from build123d import *

# Parameters (mm, degrees)
ESQUISSE1_W        = 400
ESQUISSE1_H        = 400
ESQUISSE1_R        = 150
BOSS_EXTRU_1_DEPTH = 5
BOSS_EXTRU_2_START = -5
BOSS_EXTRU_2_DEPTH = 5
BOSS_EXTRU_4_START = -5
BOSS_EXTRU_4_DEPTH = 5


with BuildPart() as part:
    # Esquisse1 → Boss.-Extru.1 (new body)
    with BuildSketch(Plane.XY):
        Rectangle(ESQUISSE1_W, ESQUISSE1_H)
        Circle(ESQUISSE1_R, mode=Mode.SUBTRACT)
    extrude(amount=BOSS_EXTRU_1_DEPTH)

    # Esquisse2 → Boss.-Extru.2 (add)
    with BuildSketch(Plane.XY.offset(5).offset(BOSS_EXTRU_2_START)):
        with BuildLine():
            ThreePointArc((-66.275928016, -134.564116188), (17.903034415, -98.409800426), (109.421717045, -102.600622995))
            ThreePointArc((109.421717045, -102.600622995), (26.84783049, -147.57775577), (-66.275928016, -134.564116188))
        make_face()
    extrude(amount=BOSS_EXTRU_2_DEPTH)

    # Esquisse5 → Boss.-Extru.4 (add)
    with BuildSketch(Plane.XY.offset(5).offset(BOSS_EXTRU_4_START)):
        with BuildLine():
            Line((-18.866345265, -83.351919662), (-20.37407273, -83.74523987))
            add(Edge.make_bspline(
                [(-20.37407273, -83.74523987), (-18.831576298, -81.763764071), (-16.735860805, -80.369241418)],
                knots=[0, 0, 0, 1, 1, 1], degree=2))
            add(Edge.make_bspline(
                [(-16.735860805, -80.369241418), (-19.802386047, -79.615782741), (-22.460949022, -81.422874022)],
                knots=[0, 0, 0, 1, 1, 1], degree=2))
            Line((-22.460949022, -81.422874022), (-21.677782316, -79.558228062))
            add(Edge.make_bspline(
                [(-21.677782316, -79.558228062), (-24.26181325, -80.142481289), (-25.822525036, -82.262094558)],
                knots=[0, 0, 0, 1, 1, 1], degree=2))
            Line((-25.822525036, -82.262094558), (-25.822525036, -81.483648674))
            add(Edge.make_bspline(
                [(-25.822525036, -81.483648674), (-28.351333433, -83.259460466), (-29.053841556, -86.259564776)],
                knots=[0, 0, 0, 1, 1, 1], degree=2))
            Line((-29.053841556, -86.259564776), (-29.496527169, -84.468232294))
            add(Edge.make_bspline(
                [(-29.496527169, -84.468232294), (-30.385431001, -86.732906367), (-30.059960229, -91.485672478), (-26.658406188, -96.353832625), (-25.176717422, -99.770059496), (-25.385021469, -101.387375039)],
                knots=[0, 0, 0, 0, 0.406589929, 0.730891559, 1, 1, 1, 1], degree=3))
            add(Edge.make_bspline(
                [(-25.385021469, -101.387375039), (-26.802377477, -98.375380833), (-29.974054698, -97.359243335)],
                knots=[0, 0, 0, 1, 1, 1], degree=2))
            Line((-29.974054698, -97.359243335), (-32.122945451, -94.451438986))
            Line((-32.122945451, -94.451438986), (-30.527430237, -94.731681614))
            Line((-30.527430237, -94.731681614), (-31.880933057, -92.683136884))
            Line((-31.880933057, -92.683136884), (-33.497007064, -90.538320458))
            Line((-33.497007064, -90.538320458), (-32.581262202, -90.538320458))
            Line((-32.581262202, -90.538320458), (-33.613359396, -89.007007118))
            Line((-33.613359396, -89.007007118), (-36.217522242, -87.522991031))
            Line((-36.217522242, -87.522991031), (-34.976085707, -87.301815556))
            Line((-34.976085707, -87.301815556), (-36.099822643, -86.512016486))
            add(Edge.make_bspline(
                [(-36.099822643, -86.512016486), (-39.217212358, -85.557948169), (-40.645373336, -82.598959987)],
                knots=[0, 0, 0, 1, 1, 1], degree=2))
            add(Edge.make_bspline(
                [(-40.645373336, -82.598959987), (-39.03359815, -80.653112191), (-34.181178142, -77.850858673), (-32.852259513, -72.300227157), (-30.904376568, -70.414710171)],
                knots=[0, 0, 0, 0, 0.487449068, 1, 1, 1, 1], degree=3))
            Line((-30.904376568, -70.414710171), (-31.646902368, -69.877944585))
            Line((-31.646902368, -69.877944585), (-29.609451058, -70.166012753))
            Line((-29.609451058, -70.166012753), (-30.237434638, -69.028235393))
            Line((-30.237434638, -69.028235393), (-32.249484484, -67.755751936))
            Line((-32.249484484, -67.755751936), (-30.841080327, -67.755751936))
            Line((-30.841080327, -67.755751936), (-32.866048633, -66.115953665))
            Line((-32.866048633, -66.115953665), (-32.122945451, -65.705806115))
            Line((-32.122945451, -65.705806115), (-34.976085707, -62.978029277))
            add(Edge.make_bspline(
                [(-34.976085707, -62.978029277), (-34.102733297, -60.394072595), (-33.737935509, -52.117151528), (-39.05614256, -45.345642181), (-42.031693147, -41.294166441)],
                knots=[0, 0, 0, 0, 0.344230119, 1, 1, 1, 1], degree=3))
            Line((-42.031693147, -41.294166441), (-43.185854427, -41.294166441))
            Line((-43.185854427, -41.294166441), (-44.096631121, -43.298315386))
            add(Edge.make_bspline(
                [(-44.096631121, -43.298315386), (-45.231201574, -46.338252094), (-48.330686607, -50.268996334), (-48.834287807, -55.064729459), (-49.3765867, -56.376310655)],
                knots=[0, 0, 0, 0, 0.699335622, 1, 1, 1, 1], degree=3))
            add(Edge.make_bspline(
                [(-49.3765867, -56.376310655), (-53.035018211, -56.310042975), (-56.717874117, -57.429335725), (-59.748293818, -59.471450261)],
                knots=[0, 0, 0, 0, 1, 1, 1, 1], degree=3))
            add(Edge.make_bspline(
                [(-59.748293818, -59.471450261), (-61.730136737, -57.382399641), (-67.02409653, -54.780846239), (-72.769327351, -53.559543058), (-75.231721344, -51.783479704)],
                knots=[0, 0, 0, 0, 0.486790351, 1, 1, 1, 1], degree=3))
            Line((-75.231721344, -51.783479704), (-76.616603351, -52.328679392))
            Line((-76.616603351, -52.328679392), (-76.910233832, -52.974808375))
            add(Edge.make_bspline(
                [(-76.910233832, -52.974808375), (-76.187929468, -60.035339336), (-73.946183278, -67.404517716), (-68.30337696, -72.2011591)],
                knots=[0, 0, 0, 0, 1, 1, 1, 1], degree=3))
            Line((-68.30337696, -72.2011591), (-70.400668481, -77.268167724))
            Line((-70.400668481, -77.268167724), (-70.400668481, -78.023881232))
            Line((-70.400668481, -78.023881232), (-69.598297697, -77.87343671))
            Line((-69.598297697, -77.87343671), (-70.283656075, -80.205357998))
            Line((-70.283656075, -80.205357998), (-70.283656075, -80.865611092))
            Line((-70.283656075, -80.865611092), (-69.087412979, -80.205357998))
            Line((-69.087412979, -80.205357998), (-69.721157599, -81.884742883))
            Line((-69.721157599, -81.884742883), (-69.721157599, -83.255626103))
            Line((-69.721157599, -83.255626103), (-68.175660205, -82.19091787))
            Line((-68.175660205, -82.19091787), (-68.497334605, -83.74523987))
            Line((-68.497334605, -83.74523987), (-67.932636696, -83.958338287))
            add(Edge.make_bspline(
                [(-67.932636696, -83.958338287), (-65.874908009, -84.443832393), (-61.558935468, -86.72875783), (-56.654005751, -85.685370072), (-54.241439725, -85.638363098)],
                knots=[0, 0, 0, 0, 0.460172434, 1, 1, 1, 1], degree=3))
            add(Edge.make_bspline(
                [(-54.241439725, -85.638363098), (-53.550315945, -86.398092796), (-52.60563993, -89.456662165), (-54.737135432, -92.036882428), (-55.189595432, -93.773610113)],
                knots=[0, 0, 0, 0, 0.354288348, 1, 1, 1, 1], degree=3))
            Line((-55.189595432, -93.773610113), (-54.110273533, -93.367103715))
            Line((-54.110273533, -93.367103715), (-55.189595432, -95.920472028))
            Line((-55.189595432, -95.920472028), (-55.189595432, -98.016520642))
            Line((-55.189595432, -98.016520642), (-54.649934483, -97.457574345))
            Line((-54.649934483, -97.457574345), (-54.919764957, -99.950163153))
            Line((-54.919764957, -99.950163153), (-54.649934483, -102.693612698))
            Line((-54.649934483, -102.693612698), (-53.518777052, -101.045082478))
            Line((-53.518777052, -101.045082478), (-53.518777052, -104.785031634))
            add(Edge.make_bspline(
                [(-53.518777052, -104.785031634), (-54.784378844, -106.350541416), (-55.393137974, -111.388492438), (-52.283724717, -115.433656634), (-50.152818663, -117.095817906)],
                knots=[0, 0, 0, 0, 0.414653077, 1, 1, 1, 1], degree=3))
            Line((-50.152818663, -117.095817906), (-50.152818663, -116.458357954))
            Line((-50.152818663, -116.458357954), (-48.056952099, -118.529915166))
            add(Edge.make_bspline(
                [(-48.056952099, -118.529915166), (-48.859432542, -119.698539939), (-48.350236289, -121.515764764), (-47.092095427, -122.118637282)],
                knots=[0, 0, 0, 0, 1, 1, 1, 1], degree=3))
            ThreePointArc((-47.092095427, -122.118637282), (-31.094519185, -113.8787786), (-14.435031904, -107.075896838))
            add(Edge.make_bspline(
                [(-14.435031904, -107.075896838), (-11.14848124, -103.537505901), (-12.000082878, -93.183121296), (-20.698698174, -88.228707084), (-18.866345265, -83.351919662)],
                knots=[0, 0, 0, 0, 0.525387835, 1, 1, 1, 1], degree=3))
        make_face()
    extrude(amount=BOSS_EXTRU_4_DEPTH)


solid = part.part
Design review of the part built by this model. Coordinates are the model's own, in mm. Coordinates: 2 decimals unless noted, no trailing zeros. Loops run counter-clockwise (first coordinate to the right, second up) from the corner with the lowest first, then second, coordinate; pieces in that order, holes last. Notation, with made-up numbers: (-3.75, 86.25) -> (7.25, 86.25) arc R8 cw to (7.25, 97.25) -> close; hole circle Ø1 at (85, 87). An arc over 180 degrees is marked (long way). Use a Markdown table: item, result. Add a question column.
Item 1: We need section A-A, the plane y = 0. Write out the cut boundary in (x, z).
Item 2: The part is to be moulded in two halves that separate along Y. For faces 1 (the flat face through (-47, -86, 0)), 2 (the cylindrical face through (-56.99, -128.16, 2.46)), 3 (the cylindrical face through (46.27, -95.27, 2.46)), say which applies: +Y half, -Y half, draft (parallel to the pull), parting line (faces both ways), or undercut.
Item 3: Wall thickness on L1, parallel to X at y = 0, z = 2.3; L2, parallel to Y at x = -71, z = 4.7; L3, parallel to Y at x = -65, z = 2.55: over which ranges is each line inside the solid? List them lowest first. Write a range as from..to.
Item 4: We need section B-B, the plane x = 129.5. Write out the cut boundary in (y, z), and give its area (3 significant figures).
Numbers:
| question | item | result |
|---|---|---|
| 1 | outline | (-200, 0) -> (-150, 0) -> (-150, 5) -> (-200, 5) -> close; (150, 0) -> (200, 0) -> (200, 5) -> (150, 5) -> close |
| 2 | face 1 | draft |
| 2 | face 2 | undercut |
| 2 | face 3 | undercut |
| 3 | L1 | x = -200..-150, 150..200 |
| 3 | L2 | y = -200..-132.13, -69.42..-53.86, 132.13..200 |
| 3 | L3 | y = -200..-133.64, -84.91..-55.95, 135.19..200 |
| 4 | outline | (-200, 0) -> (-75.7, 0) -> (-75.7, 5) -> (-200, 5) -> close; (75.7, 0) -> (200, 0) -> (200, 5) -> (75.7, 5) -> close |
| 4 | area | 1,240 mm^2 |
